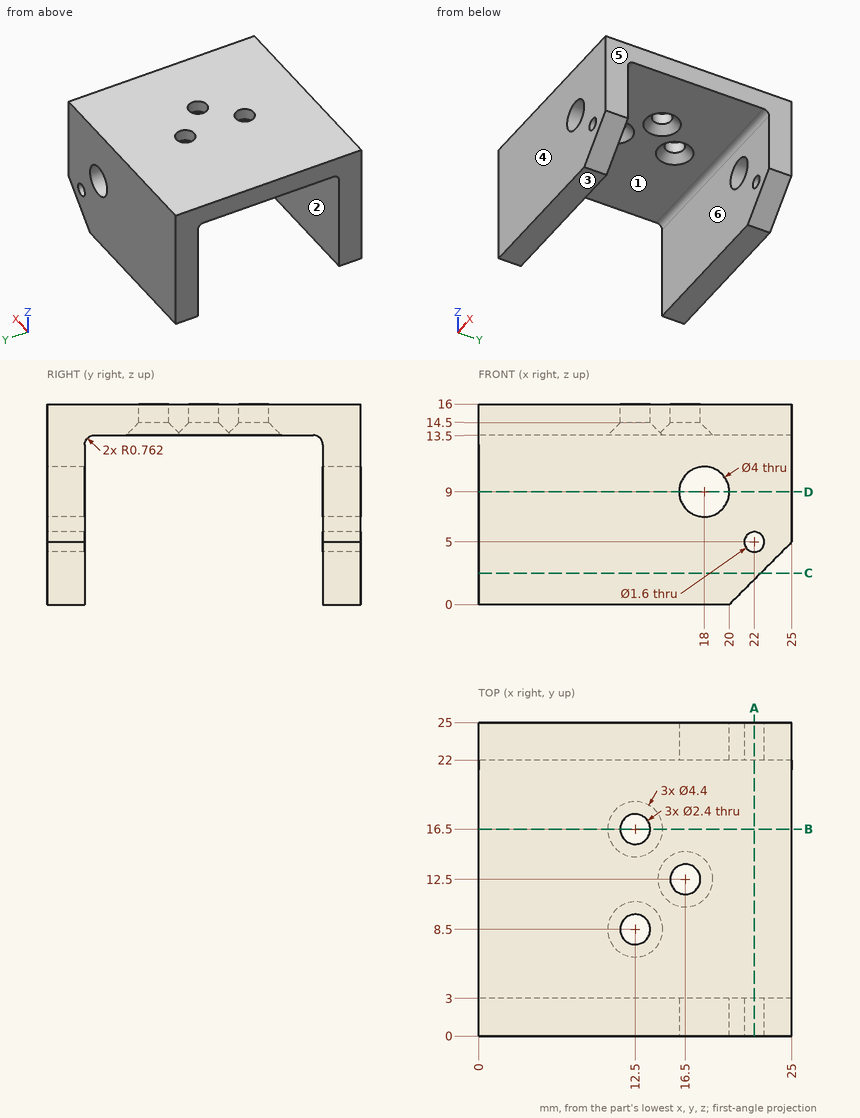
Input: dimensioned drawing with shaded views. Units: mm. Origin: part minimum x, y, z. A direction names the side the tool comes from. Coordinates: 2 decimals unless noted, no trailing zeros. Order: outer loops, then holes, each group sorted by start corner. A loop starts at its lowest first (then second) coordinate and runs counter-clockwise, first axis right, second up. Notation, with made-up numbers: (28, 66.25) - (65, 66.25) arc R27 ccw to (65, 84.25) - close; hole circle Ø6 at (-34.5, -24). An arc over 180 degrees is marked (long way). Return JSON: item names as keys, results as strings. Group by question number.
1. Cut plane B-B (y = 16.5). Output: boundary loops of the cut face in (x, z).
2. Cut plane D-D (z = 9). Output: boundary loops of the cut face in (x, y), plus the area to 3 significant figures.
3. Pull-direction query (Y, two-part tool) for the marked faces 1, 2, 3 and 4; classes: pulls with the +Y half, pulls with the -Y half, needs draft (parallel to the pull), parting line crosses it, or undercut.
4. Set-up query: the marked faces 5 and 6. Return all of +Z, -Z, +X, -X, +Y, -Y with unobstructed straight access to the full face (end or side cutting, diameter ignored); none if empty.
5. Material intervals for line 1 along Y through (x, z) = (8, 2.5); line 2 along Z through (x, y) = (18, 23.4); line 3 along Y through (x, z) = (12.5, 15.05), sorted ascending. Write a range as [from, to].
6. Cut plane A-A (x = 22). Output: boundary loops of the cut face in (y, z), plus the area to 3 significant figures.
7. Pin query (flat end, axial travel): pin 1 (2 mm diameter, centred on x = 22, z = 5, fed in from +Y); pin 2 (4 mm diameter, centred on x = 12.5, y = 8.5, fed in from -Z); pin 3 (5 mm diameter, centred on x = 6, y = 9, fed in from -Z). Return the tip coordinate at first contact, or that it passes through.
8. Cut plane C-C (z = 2.5). Output: boundary loops of the cut face in (x, y).
Resolved:
{
 "1": {"outline": "(0, 13.5) - (10.3, 13.5) - (11.3, 14.5) - (11.3, 16) - (0, 16) - close; (13.7, 14.5) - (14.7, 13.5) - (25, 13.5) - (25, 16) - (13.7, 16) - close"},
 "2": {"outline": "(0, 0) - (16, 0) - (16, 3) - (0, 3) - close; (0, 22) - (16, 22) - (16, 25) - (0, 25) - close; (20, 0) - (25, 0) - (25, 3) - (20, 3) - close; (20, 22) - (25, 22) - (25, 25) - (20, 25) - close", "area": "126 mm²"},
 "3": {"face 1": "undercut", "face 2": "undercut", "face 3": "needs draft", "face 4": "pulls with the -Y half"},
 "4": {"face 5": "+Z, -Z, +X, +Y, -Y", "face 6": "-Z, +X, -X"},
 "5": {"line 1": "y = [0, 3], [22, 25]", "line 2": "z = [0, 7], [11, 16]", "line 3": "y = [0, 7.3], [9.7, 15.3], [17.7, 25]"},
 "6": {"outline": "(0, 2) - (3, 2) - (3, 4.2) - (0, 4.2) - close; (0, 5.8) - (3, 5.8) - (3, 12.74) arc R0.76 cw to (3.76, 13.5) - (21.24, 13.5) arc R0.76 cw to (22, 12.74) - (22, 5.8) - (25, 5.8) - (25, 16) - (0, 16) - close; (22, 2) - (25, 2) - (25, 4.2) - (22, 4.2) - close", "area": "122 mm²"},
 "7": {"pin 1": "stops at y = 25", "pin 2": "stops at z = 13.7", "pin 3": "stops at z = 13.5"},
 "8": {"outline": "(0, 0) - (22.5, 0) - (22.5, 3) - (0, 3) - close; (0, 22) - (22.5, 22) - (22.5, 25) - (0, 25) - close"}
}
